from build123d import *

# Parameters (mm, degrees)
SKETCH_2_R          = 15
CUT_EXTRUDE_1_DEPTH = 78.614431648
SKETCH_3_R          = 35
CUT_EXTRUDE_2_DEPTH = 3
SKETCH_4_R          = 4.5
CUT_EXTRUDE_3_DEPTH = 78.614431648


with BuildPart() as part:
    # 草图1 → 旋转1 (revolve)
    with BuildSketch(Plane(origin=(0, 0, 0), x_dir=(1, 0, 0), z_dir=(0, 1, 0)), mode=Mode.PRIVATE) as revolve_1_sk:
        Polygon((0, 0), (50, 0), (50, -12), (25, -12), (25, -32), (0, -32), align=None)
    revolve(revolve_1_sk.sketch.rotate(Axis((0, 0, 0), (0, 0, 1)), 180), axis=Axis((0, 0, 0), (0, 0, 1)))

    # 草图2 → 切除-拉伸1 (cut, through all)
    with BuildSketch(Plane.XY):
        Circle(SKETCH_2_R)
    extrude(amount=CUT_EXTRUDE_1_DEPTH, mode=Mode.SUBTRACT)

    # 草图3 → 切除-拉伸2 (cut)
    with BuildSketch(Plane.XY):
        Circle(SKETCH_3_R)
    extrude(amount=CUT_EXTRUDE_2_DEPTH, mode=Mode.SUBTRACT)

    # 草图4 → 切除-拉伸3 (cut, through all)
    with BuildSketch(Plane.XY.offset(32)):
        with Locations((40, 0)):
            Circle(SKETCH_4_R)
        with Locations((20, 34.641016)):
            Circle(SKETCH_4_R)
        with Locations((-20, 34.641016)):
            Circle(SKETCH_4_R)
        with Locations((-40, 0)):
            Circle(SKETCH_4_R)
        with Locations((-20, -34.641016)):
            Circle(SKETCH_4_R)
        with Locations((20, -34.641016)):
            Circle(SKETCH_4_R)
    extrude(amount=-CUT_EXTRUDE_3_DEPTH, mode=Mode.SUBTRACT)


solid = part.part
Part model, mm, in its own coordinate system. A direction names the side the tool comes from. Coordinates: 2 decimals unless noted, no trailing zeros. Write each loop counter-clockwise with the first axis right and the second up, starting at its lowest first coordinate (ties: lowest second). Pieces come first, ordered by that corner, then holes. Notation, with made-up numbers: (51.25, 26.5) - (106.25, 26.5) arc R4 cw to (106.25, 30.5) - close; hole circle Ø4 at (37.25, 35). An arc over 180 degrees is marked (long way). Put each result on its own line as item: value.
1. Band-saw the part on C-C (z = 4.5). Write the cut outline in (x, y).
Final values:
outline: circle Ø100 at (0, 0); hole circle Ø9 at (-40, 0); hole circle Ø9 at (-20, -34.64); hole circle Ø9 at (-20, 34.64); hole circle Ø30 at (0, 0); hole circle Ø9 at (20, -34.64); hole circle Ø9 at (20, 34.64); hole circle Ø9 at (40, 0)
2. Two-plate mould, pull along Y, no slides. Class faces 4 (the cylindrical face through (19.02, 30.25, 6.08)), 5 (the cylindrical face through (19.024, -39.034, 6.084)), 6 (the flat face through (22.9, 10.4, 12)), 7 (the cylindrical face through (-47.69, -15.02, 6.08)): +Y half, -Y half, draft (parallel to the pull), parting line (faces both ways), or undercut.
Final values:
face 4: undercut
face 5: undercut
face 6: draft
face 7: parting line
3. Band-saw the part on B-B (x = 0). Write the cut outline in (y, z).
Final values:
outline: (-50, 0) - (-35, 0) - (-35, 3) - (-15, 3) - (-15, 32) - (-25, 32) - (-25, 12) - (-50, 12) - close; (15, 3) - (35, 3) - (35, 0) - (50, 0) - (50, 12) - (25, 12) - (25, 32) - (15, 32) - close
4. Band-saw the part on D-D (x = -20). Write the cut outline in (y, z), then the cut area to 3 significant figures.
Final values:
outline: (-45.83, 0) - (-39.14, 0) - (-39.14, 12) - (-45.83, 12) - close; (-30.14, 0) - (-28.72, 0) - (-28.72, 3) - (28.72, 3) - (28.72, 0) - (30.14, 0) - (30.14, 12) - (15, 12) - (15, 32) - (-15, 32) - (-15, 12) - (-30.14, 12) - close; (39.14, 0) - (45.83, 0) - (45.83, 12) - (39.14, 12) - close
area: 1,310 mm²
5. Probe line 1 along Y through (x, z) = (0, 5); line 2 along Z through (x, y) = (35, 28.5); line 3 along Z through (x, y) = (-24, 3). List the from-to ranges inside material, lowest first. Write a range as [from, to].
Final values:
line 1: y = [-50, -15], [15, 50]
line 2: z = [0, 12]
line 3: z = [3, 32]
6. Band-saw the part on A-A (y = 0). Write the cut outline in (x, z), then the cut area to 3 significant figures.
Final values:
outline: (-50, 0) - (-44.5, 0) - (-44.5, 12) - (-50, 12) - close; (-35.5, 0) - (-35, 0) - (-35, 3) - (-15, 3) - (-15, 32) - (-25, 32) - (-25, 12) - (-35.5, 12) - close; (15, 3) - (35, 3) - (35, 0) - (35.5, 0) - (35.5, 12) - (25, 12) - (25, 32) - (15, 32) - close; (44.5, 0) - (50, 0) - (50, 12) - (44.5, 12) - close
area: 904 mm²
7. Flat gauge pins, fed straight in: pin 1 Ø3 at (x, y) = (28.5, -1.5) entering from -Z; pin 2 Ø8 at (y, z) = (-18.5, 3.5) entering from -X; pin 3 Ø11.5 at (x, y) = (20, -34.64) entering from +Z. Where does each tip first touch, or does it go through?
Final values:
pin 1: stops at z = 3
pin 2: stops at x = -47.85
pin 3: stops at z = 12
8. 3-axis set-ups, long thin cutter, end or side, ignore diameter. For faces 1 (the cylindrical face through (-23.846, -7.509, 22.14)), 2 (the cylindrical face through (-28, -21, 1)), 3 (the flat face through (-11, 11, 32)): which of +Z, -Z, +X, -X, +Y, -Y reach the whole face in a straight line?
Final values:
face 1: +Z
face 2: -Z
face 3: +Z, +X, -X, +Y, -Y
